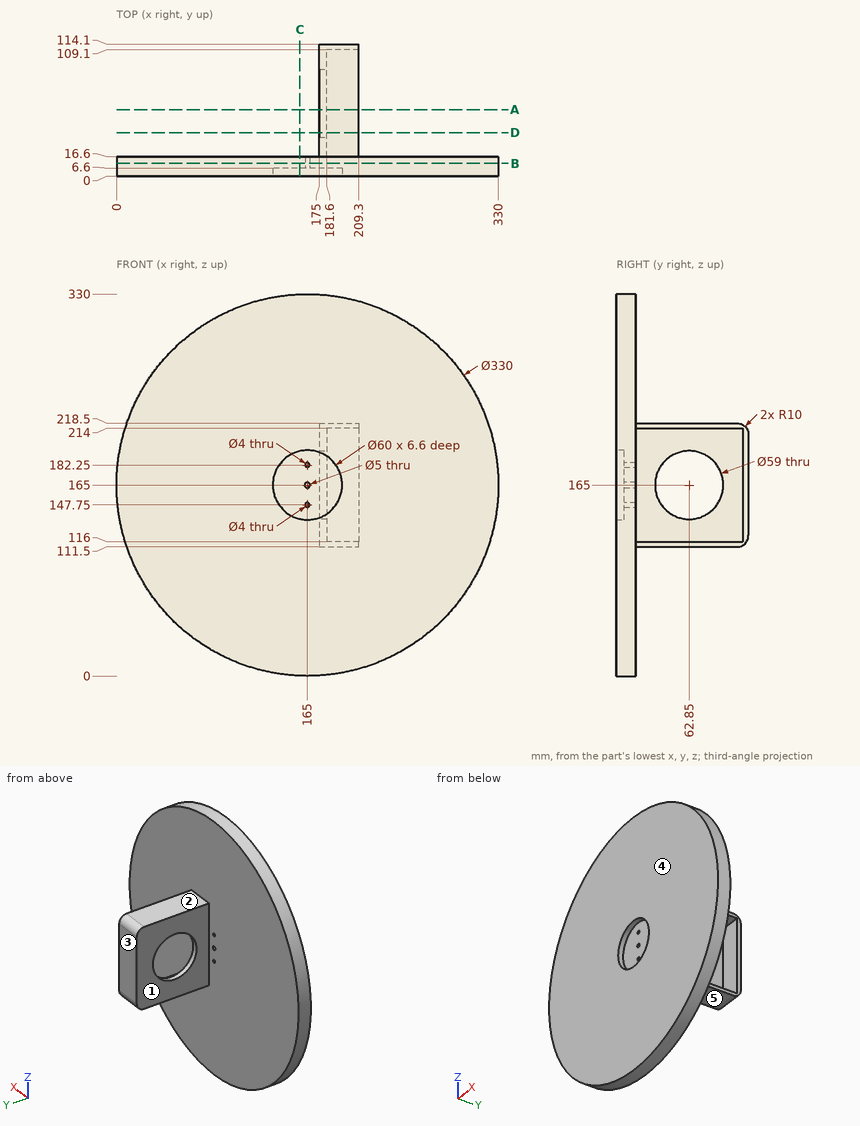
The figure shows three views and two pictorial views of one solid part (mm, origin at its lowest corner). Answer the questions. A direction names the side the tool comes from. Round coordinates to 2 decimals unless told otherwise and drop trailing zeros. Write each loop counter-clockwise with the first axis right and the second up, starting at its lowest first coordinate (ties: lowest second). Pieces come first, ordered by that corner, then holes. Notation, with made-up numbers: M -6,37 L 22,37 A17 ccw 22,53 Z; hole C 17,25.5 d6. An arc over 180 degrees is marked long. Write each question's results on one line, items separated by ' | '. Start each with the question number.
(1) The part is cut by section B-B, the plane y = 11. Write down the section's boundary in (x, z), and give its area (3 significant figures).
(2) The part is cut by section A-A, the plane y = 57.5. Write down the section's boundary in (x, z).
(3) The part is cut by section D-D, the plane y = 37.5. Write down the section's boundary in (x, z).
(4) For the marked faces 1, 2, 3, 4 and 5, determine the directions among +Z, -Z, +X, -X, +Y, -Y from which every point of the face is accessible in a straight line to the end or side of a thin tool.
(5) Each of these flat-tipped pins is pushed along its axis until it touches: P1, Ø3.5, axis at x = 165, z = 147.75, coming from the -Y side; P2, Ø1, axis at y = 56, z = 117.5, coming from the -X side; P3, Ø1.5, axis at x = 184.5, z = 179, coming from the -Y side; P4, Ø8, axis at x = 186, z = 112.5, coming from the +Y side. Where does it stop, or does it pass through?
(6) Find the intervals of material crossed by line 1 (Z direction, x = 176, y = 62); line 2 (Z direction, x = 186.5, y = 47); line 3 (X direction, y = 11.5, z = 165), in increasing order.
(7) The part is cut by section C-C, the plane x = 158.5. Write down the section's boundary in (y, z), and give its area (3 significant figures).
Worked answers:
1) outline: C 165,165 d330; hole C 165,165 d5; hole C 165,147.75 d4; hole C 165,182.25 d4 | area: 85,500 mm²
2) outline: M 175,111.5 L 209.3,111.5 L 209.3,116 L 181.6,116 L 181.6,135.99 L 175,135.99 Z; M 175,194.01 L 181.6,194.01 L 181.6,214 L 209.3,214 L 209.3,218.5 L 175,218.5 Z
3) outline: M 175,111.5 L 209.3,111.5 L 209.3,116 L 181.6,116 L 181.6,149.91 L 175,149.91 Z; M 175,180.09 L 181.6,180.09 L 181.6,214 L 209.3,214 L 209.3,218.5 L 175,218.5 Z
4) face 1: +Z, -Z, -X, +Y | face 2: +Z, +X, -X, +Y | face 3: +Z, -Z, +X, -X, +Y | face 4: +Z, -Z, +X, -X, -Y | face 5: -Z, +X, -X, +Y
5) P1: passes through | P2: stops at x = 175 | P3: stops at y = 6.6 | P4: stops at y = 112.76
6) line 1: z = 111.5 to 135.51, 194.49 to 218.5 | line 2: z = 111.5 to 116, 214 to 218.5 | line 3: x = 0 to 162.5, 167.5 to 330
7) outline: M 0,0.13 L 16.6,0.13 L 16.6,329.87 L 0,329.87 L 0,194.29 L 6.6,194.29 L 6.6,135.71 L 0,135.71 Z | area: 5,090 mm²
